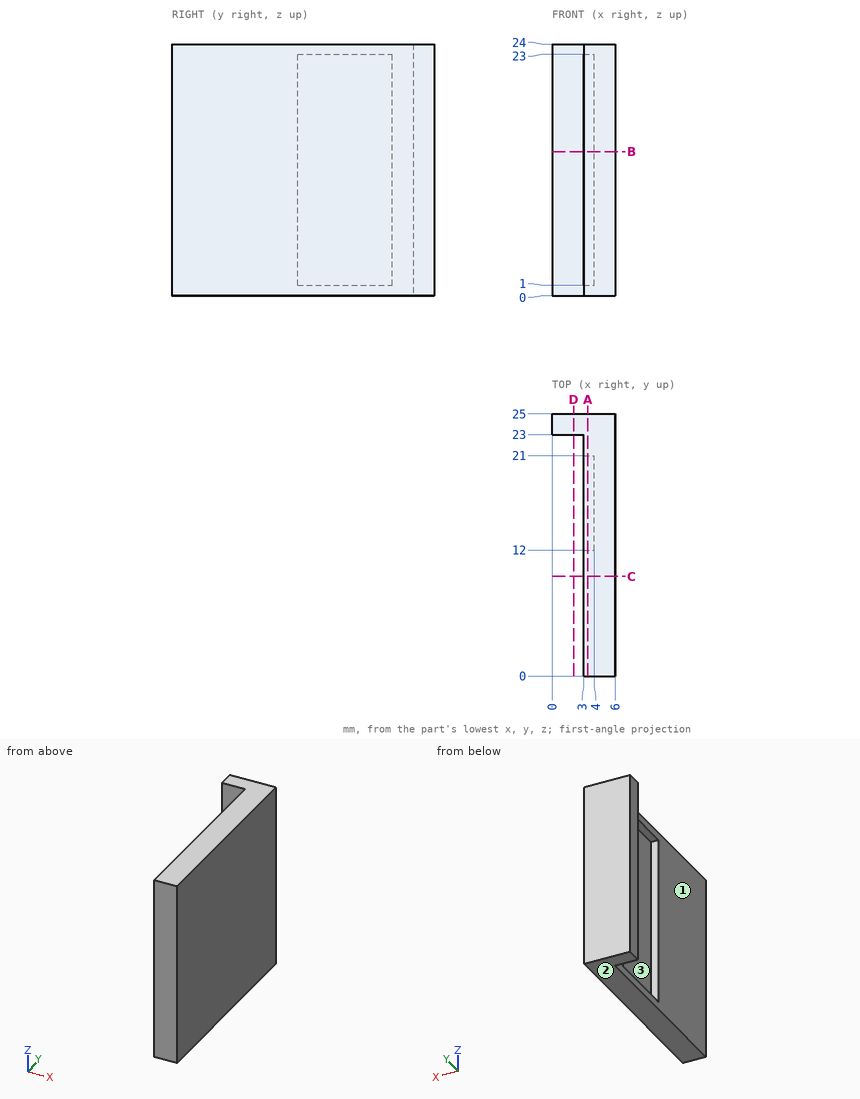
Input: dimensioned drawing with shaded views. Units: mm. Origin: part minimum x, y, z. Coordinates: 2 decimals unless noted, no trailing zeros. Loops run counter-clockwise (first coordinate to the right, second up) from the corner with the lowest first, then second, coordinate; pieces in that order, holes last. Notation, with made-up numbers: M 76.5,-39 L 120.5,-39 A20 ccw 120.5,-14 Z; hole C -38,-21 d9. An arc over 180 degrees is marked long. One line per item, written item: value. Start each with the question number.
1) Material intervals for L1, parallel to Y at x = 3.9, z = 13.25; L2, parallel to Y at x = 1.7, z = 18.5; L3, parallel to X at y = 1, z = 21, sorted ascending. Write a range as from..to.
2) Cut plane C-C (y = 9.5). Return loops of the section in (x, z).
3) Cut plane D-D (x = 2.05). Return loops of the section in (y, z).
4) Draft query along Z for the marked faces 1, 2 and 3. Return one class per face: released by +Z, released by -Z, zero draft, split by the parting line, or undercut.
5) Cut plane A-A (x = 3.4). Return loops of the section in (y, z), then the cut area to 3 significant figures.
6) Pin query (flat end, axial travel): P1, Ø0.9, axis at x = 2, z = 15.5, coming from the -Y side; P2, Ø7, axis at y = 17, z = 14.5, coming from the -X side; P3, Ø10, axis at y = 11, z = 10.5, coming from the -X side; P4, Ø0.5, axis at x = 3.5, y = 15.5, coming from the -Z side. Return the tip coordinate at first contact, or that it passes through.
7) Cut plane B-B (z = 13.75). Return loops of the section in (x, y).
Evaluation:
1. L1: 0..12, 21..25
1. L2: 23..25
1. L3: 3..6
2. outline: M 3,0 L 6,0 L 6,24 L 3,24 Z
3. outline: M 23,0 L 25,0 L 25,24 L 23,24 Z
4. face 1: zero draft
4. face 2: released by -Z
4. face 3: undercut
5. outline: M 0,0 L 25,0 L 25,24 L 0,24 Z; hole M 12,1 L 21,1 L 21,23 L 12,23 Z
5. area: 402 mm^2
6. P1: y = 23
6. P2: x = 4
6. P3: x = 3
6. P4: z = 0
7. outline: M 0,23 L 3,23 L 3,21 L 4,21 L 4,12 L 3,12 L 3,0 L 6,0 L 6,25 L 0,25 Z
